```python
from build123d import *

# Parameters (mm, degrees)
BOSS_EXTRUDE1_DEPTH            = 25
SKETCH2_R                      = 2.6
SKETCH2_R_2                    = 1.55
BOSS_EXTRUDE3_DEPTH            = 5
CUT_EXTRUDE1_REACH             = 98.604
CUT_EXTRUDE1_DIRECTION_2_DEPTH = 97.603907966
CUT_EXTRUDE2_REACH             = 98.604
CUT_EXTRUDE2_DIRECTION_2_DEPTH = 97.603907966
FILLET1_R                      = 2
SKETCH6_R                      = 2.6
BOSS_EXTRUDE4_DEPTH            = 1


with BuildPart() as part:
    # Sketch1 → Boss-Extrude1 (new body)
    with BuildSketch(Plane(origin=(0, 0, 0), x_dir=(1, 0, 0), z_dir=(0, 1, 0))):
        Polygon((-13.5, 0), (0, 83.718518379), (13.5, 0), (14.487246657, 0.15919811), (0, 90), (-14.487246657, 0.15919811), align=None)
    extrude(amount=BOSS_EXTRUDE1_DEPTH)

    # Sketch2 → Boss-Extrude3 (add)
    # profile 1 of 8: a face of its own
    with BuildSketch(Plane(origin=(0, 0, 0), x_dir=(1, 0, 0), z_dir=(0, 1, 0))):
        with Locations((11.920405349, -0.254716975)):
            Circle(SKETCH2_R)
        with Locations(Location((11.920405349, -0.254716975, 0), (0, 0, 270))):
            Circle(SKETCH2_R_2, mode=Mode.SUBTRACT)
    # profile 2 of 8: a face of its own
    with BuildSketch(Plane(origin=(0, 0, 0), x_dir=(1, 0, 0), z_dir=(0, 1, 0))):
        with Locations((9.373235594, 15.541229537)):
            Circle(SKETCH2_R)
        with Locations(Location((9.373235594, 15.541229537, 0), (0, 0, 270))):
            Circle(SKETCH2_R_2, mode=Mode.SUBTRACT)
    # profile 3 of 8: a face of its own
    with BuildSketch(Plane(origin=(0, 0, 0), x_dir=(1, 0, 0), z_dir=(0, 1, 0))):
        with Locations((6.826065839, 31.33717605)):
            Circle(SKETCH2_R)
        with Locations(Location((6.826065839, 31.33717605, 0), (0, 0, 270))):
            Circle(SKETCH2_R_2, mode=Mode.SUBTRACT)
    # profile 4 of 8: a face of its own
    with BuildSketch(Plane(origin=(0, 0, 0), x_dir=(1, 0, 0), z_dir=(0, 1, 0))):
        with Locations((4.278896085, 47.133122563)):
            Circle(SKETCH2_R)
        with Locations(Location((4.278896085, 47.133122563, 0), (0, 0, 270))):
            Circle(SKETCH2_R_2, mode=Mode.SUBTRACT)
    # profile 5 of 8: a face of its own
    with BuildSketch(Plane(origin=(0, 0, 0), x_dir=(1, 0, 0), z_dir=(0, 1, 0))):
        with Locations((-4.278896085, 47.133122563)):
            Circle(SKETCH2_R)
        with Locations(Location((-4.278896085, 47.133122563, 0), (0, 0, 90))):
            Circle(SKETCH2_R_2, mode=Mode.SUBTRACT)
    # profile 6 of 8: a face of its own
    with BuildSketch(Plane(origin=(0, 0, 0), x_dir=(1, 0, 0), z_dir=(0, 1, 0))):
        with Locations((-6.826065839, 31.33717605)):
            Circle(SKETCH2_R)
        with Locations(Location((-6.826065839, 31.33717605, 0), (0, 0, 90))):
            Circle(SKETCH2_R_2, mode=Mode.SUBTRACT)
    # profile 7 of 8: a face of its own
    with BuildSketch(Plane(origin=(0, 0, 0), x_dir=(1, 0, 0), z_dir=(0, 1, 0))):
        with Locations((-9.373235594, 15.541229537)):
            Circle(SKETCH2_R)
        with Locations(Location((-9.373235594, 15.541229537, 0), (0, 0, 90))):
            Circle(SKETCH2_R_2, mode=Mode.SUBTRACT)
    # profile 8 of 8: a face of its own
    with BuildSketch(Plane(origin=(0, 0, 0), x_dir=(1, 0, 0), z_dir=(0, 1, 0))):
        with Locations((-11.920405349, -0.254716975)):
            Circle(SKETCH2_R)
        with Locations(Location((-11.920405349, -0.254716975, 0), (0, 0, 90))):
            Circle(SKETCH2_R_2, mode=Mode.SUBTRACT)
    boss_extrude3 = extrude(amount=BOSS_EXTRUDE3_DEPTH)

    # Cut-Extrude1: up to this face of the body (flat: up to its plane)
    cut_extrude1_end = Plane(part.part.faces().sort_by_distance((-6.667350715, 12.850191169, -42.371798131))[0])
    # Sketch4 → Cut-Extrude1 (cut, up to the picked face)
    with BuildSketch(Plane(origin=(0.342144515, 0, 2.121765321), x_dir=(0.9872466570606503, 0, -0.1591981096702188), z_dir=(0.1591981096702188, 0, 0.9872466570606503)), mode=Mode.PRIVATE) as cut_extrude1_sk1:
        Polygon((13.32782987, 5), (9.12782987, 5), (9.12782987, 1.475781549), align=None)
    cut_extrude1_tool1 = split(extrude(cut_extrude1_sk1.sketch, amount=-CUT_EXTRUDE1_REACH, mode=Mode.PRIVATE), bisect_by=cut_extrude1_end, keep=Keep.BOTH, mode=Mode.PRIVATE)
    cut_extrude1 = cut_extrude1_tool1.solids().sort_by(Axis((10.735709, 3.825261, 0.445755), (-0.1591981096702188, 0, -0.9872466570606503)))[0]
    add(cut_extrude1, mode=Mode.SUBTRACT)

    # Sketch4 → Cut-Extrude1 direction 2 (cut)
    with BuildSketch(Plane(origin=(0.342144515, 0, 2.121765321), x_dir=(0.9872466570606503, 0, -0.1591981096702188), z_dir=(0.1591981096702188, 0, 0.9872466570606503))):
        Polygon((13.32782987, 5), (9.12782987, 5), (9.12782987, 1.475781549), align=None)
    cut_extrude1_direction_2 = extrude(amount=CUT_EXTRUDE1_DIRECTION_2_DEPTH, mode=Mode.SUBTRACT)

    # Cut-Extrude2: up to this face of the body (flat: up to its plane)
    cut_extrude2_end = Plane(part.part.faces().sort_by_distance((6.667350715, 12.850191169, -42.371798131))[0])
    # Sketch5 → Cut-Extrude2 (cut, up to the picked face)
    with BuildSketch(Plane(origin=(-0.342144515, 0, 2.121765321), x_dir=(0.9872466570606502, 0, 0.15919810967021986), z_dir=(-0.15919810967021986, 0, 0.9872466570606502)), mode=Mode.PRIVATE) as cut_extrude2_sk1:
        Polygon((-9.12782987, 5), (-9.12782987, 1.475781549), (-13.32782987, 5), align=None)
    cut_extrude2_tool1 = split(extrude(cut_extrude2_sk1.sketch, amount=-CUT_EXTRUDE2_REACH, mode=Mode.PRIVATE), bisect_by=cut_extrude2_end, keep=Keep.BOTH, mode=Mode.PRIVATE)
    cut_extrude2 = cut_extrude2_tool1.solids().sort_by(Axis((-10.735709, 3.825261, 0.445755), (0.15919810967021986, 0, -0.9872466570606502)))[0]
    add(cut_extrude2, mode=Mode.SUBTRACT)

    # Sketch5 → Cut-Extrude2 direction 2 (cut)
    with BuildSketch(Plane(origin=(-0.342144515, 0, 2.121765321), x_dir=(0.9872466570606502, 0, 0.15919810967021986), z_dir=(-0.15919810967021986, 0, 0.9872466570606502))):
        Polygon((-9.12782987, 5), (-9.12782987, 1.475781549), (-13.32782987, 5), align=None)
    cut_extrude2_direction_2 = extrude(amount=CUT_EXTRUDE2_DIRECTION_2_DEPTH, mode=Mode.SUBTRACT)

    # Mirror2: Boss-Extrude3, Cut-Extrude1, Cut-Extrude1 direction 2, Cut-Extrude2, Cut-Extrude2 direction 2 across plane
    add(boss_extrude3.mirror(Plane.ZX.offset(12.5)))
    add(cut_extrude1.mirror(Plane.ZX.offset(12.5)), mode=Mode.SUBTRACT)
    add(cut_extrude1_direction_2.mirror(Plane.ZX.offset(12.5)), mode=Mode.SUBTRACT)
    add(cut_extrude2.mirror(Plane.ZX.offset(12.5)), mode=Mode.SUBTRACT)
    add(cut_extrude2_direction_2.mirror(Plane.ZX.offset(12.5)), mode=Mode.SUBTRACT)

    # Fillet1
    # the kernel refuses this fillet: 2 mm, written as the material it adds along each edge
    with BuildSketch(Plane(origin=(-19.423479942, 5, -0.955188658), x_dir=(-0.15919810967021975, 0, 0.9872466570606501), z_dir=(0.9872466570606501, 0, 0.15919810967021975))) as fillet1_piece_1_section:
        with BuildLine():
            CenterArc((FILLET1_R, -FILLET1_R), FILLET1_R, 90, 90)
            Line((0, -FILLET1_R), (0, 0))
            Line((0, 0), (FILLET1_R, 0))
        make_face()
    fillet1_piece_1 = extrude(amount=6, mode=Mode.PRIVATE)
    fillet1_piece_1 = fillet1_piece_1 & Plane(origin=(-11.920405349, 5.222362792, 0.254716975), x_dir=(1, 0, 0), z_dir=(0, -1, 0)) * Cylinder(2.6, 21, mode=Mode.PRIVATE)
    add(fillet1_piece_1)
    with BuildSketch(Plane(origin=(13.5, 5, 0), x_dir=(0, 1, 0), z_dir=(0.9872466570606502, 0, -0.15919810967021866))) as fillet1_piece_2_section:
        with BuildLine():
            CenterArc((FILLET1_R, FILLET1_R), FILLET1_R, 180, 90)
            Line((0, FILLET1_R), (0, 0))
            Line((0, 0), (FILLET1_R, 0))
        make_face()
    fillet1_piece_2 = extrude(amount=6, mode=Mode.PRIVATE)
    fillet1_piece_2 = fillet1_piece_2 & Plane(origin=(11.920405349, 5.699977741, 0.254716975), x_dir=(1, 0, 0), z_dir=(0, -1, 0)) * Cylinder(2.6, 20, mode=Mode.PRIVATE)
    add(fillet1_piece_2)
    with BuildSketch(Plane(origin=(13.5, 20, 0), x_dir=(0, -1, 0), z_dir=(0.9872466570606502, 0, -0.15919810967021866))) as fillet1_piece_3_section:
        with BuildLine():
            CenterArc((FILLET1_R, -FILLET1_R), FILLET1_R, 90, 90)
            Line((0, -FILLET1_R), (0, 0))
            Line((0, 0), (FILLET1_R, 0))
        make_face()
    fillet1_piece_3 = extrude(amount=6, mode=Mode.PRIVATE)
    fillet1_piece_3 = fillet1_piece_3 & Plane(origin=(11.920405349, 19.300022259, 0.254716975), x_dir=(1, 0, 0), z_dir=(0, 1, 0)) * Cylinder(2.6, 20, mode=Mode.PRIVATE)
    add(fillet1_piece_3)
    with BuildSketch(Plane(origin=(-19.423479942, 20, -0.955188658), x_dir=(0, -1, 0), z_dir=(0.9872466570606501, 0, 0.15919810967021975))) as fillet1_piece_4_section:
        with BuildLine():
            CenterArc((FILLET1_R, -FILLET1_R), FILLET1_R, 90, 90)
            Line((0, -FILLET1_R), (0, 0))
            Line((0, 0), (FILLET1_R, 0))
        make_face()
    fillet1_piece_4 = extrude(amount=6, mode=Mode.PRIVATE)
    fillet1_piece_4 = fillet1_piece_4 & Plane(origin=(-11.920405349, 19.777637105, 0.254716975), x_dir=(1, 0, 0), z_dir=(0, 1, 0)) * Cylinder(2.6, 21, mode=Mode.PRIVATE)
    add(fillet1_piece_4)

    # Sketch6 → Boss-Extrude4 (add)
    with BuildSketch(Plane.XZ):
        with Locations((11.920405349, 0.254716975)):
            Circle(SKETCH6_R)
        with Locations((9.373235594, -15.541229537)):
            Circle(SKETCH6_R)
        with Locations((6.826065839, -31.33717605)):
            Circle(SKETCH6_R)
        with Locations((4.278896085, -47.133122563)):
            Circle(SKETCH6_R)
        with Locations((-4.278896085, -47.133122563)):
            Circle(SKETCH6_R)
        with Locations((-6.826065839, -31.33717605)):
            Circle(SKETCH6_R)
        with Locations((-9.373235594, -15.541229537)):
            Circle(SKETCH6_R)
        with Locations((-11.920405349, 0.254716975)):
            Circle(SKETCH6_R)
    extrude(amount=-BOSS_EXTRUDE4_DEPTH)


solid = part.part
```
Geometry: final body of the model. Coordinates: model frame, mm. A direction names the side the tool comes from. Coordinates: 2 decimals unless noted, no trailing zeros. Order: outer loops, then holes, each group sorted by start corner. A loop starts at its lowest first (then second) coordinate and runs counter-clockwise, first axis right, second up. Notation, with made-up numbers: (-38.75, 2.5) -> (-3.75, 2.5) arc R16 cw to (-3.75, 13.5) -> close; hole circle Ø11 at (-13.75, -2). An arc over 180 degrees is marked (long way). Answer in a Markdown table with one row per item.
Item 1: Contact query for flat-ended pins moving along their axis: P1, Ø1.5, axis at y = 17.5, z = -14, coming from the -X side; P2, Ø4, axis at y = 5, z = -59.5, coming from the -X side; P3, Ø0.9, axis at x = 12, z = -0.5, coming from the +Y side. Output: stop coordinate, or through.
Return value:
| item | result |
|---|---|
| P1 | stops at x = -12.38 |
| P2 | stops at x = -5.24 |
| P3 | stops at y = 1 |
Item 2: Section B-B on y = 13. Output: boundary loops of the cut face in (x, z), plus the area to 3 significant figures.
Return value:
| item | result |
|---|---|
| outline | (-14.49, -0.16) -> (0, -90) -> (14.49, -0.16) -> (13.5, 0) -> (0, -83.72) -> (-13.5, 0) -> close |
| area | 176 mm² |
Item 3: Ray query, L1, parallel to Y at x = -5.25, z = -33; L2, parallel to Y at x = 4.75, z = -31; L3, parallel to X at y = 16, z = -2.5. Return the intervals inside material, ascending.
Return value:
| item | result |
|---|---|
| L1 | y = 0 to 2.57, 22.43 to 25 |
| L2 | y = 0 to 1.89, 23.11 to 25 |
| L3 | x = -14.11 to -13.1, 13.1 to 14.11 |
Item 4: Section A-A on z = -42.5. Output: boundary loops of the cut face in (x, y), plus the area to 3 significant figures.
Return value:
| item | result |
|---|---|
| outline | (-7.66, 0) -> (-6.65, 0) -> (-6.65, 25) -> (-7.66, 25) -> close; (6.65, 0) -> (7.66, 0) -> (7.66, 25) -> (6.65, 25) -> close |
| area | 50.6 mm² |
Item 5: Draft query along Y for faces 4 (the cylindrical face through (10.91, 23.1, -15.74)), 5 (the flat face through (-5.204, 2.43, -32.209)), 6 (the flat face through (-4, 1, -47)). Return one class per face: released by +Y, released by -Y, zero draft, split by the parting line, or undercut.
Return value:
| item | result |
|---|---|
| face 4 | zero draft |
| face 5 | undercut |
| face 6 | released by +Y |
Item 6: Access query for faces 1 (the flat face through (7.75, 2.43, -16.41)), 2 (the cylindrical face through (10.91, 2.52, -15.74)), 3 (the cylindrical face through (-13.95, 5.83, 0.31)). Directions: +Z, -Z, +X, -X, +Y, -Y. A direction counts if a zero-diameter tool reaches every point of the face in a straight line with its end or side. Return the directions, or none.
Return value:
| item | result |
|---|---|
| face 1 | +Z |
| face 2 | +Y |
| face 3 | +Z, -X |
Item 7: Section C-C on y = 6. Output: boundary loops of the cut face in (x, z), plus the area to 3 significant figures.
Return value:
| item | result |
|---|---|
| outline | (-14.52, 0.11) arc R2.6 ccw to (-14.49, -0.16) -> (0, -90) -> (14.49, -0.16) arc R2.6 ccw to (14.52, 0.11) -> (13.54, 0.26) -> (0, -83.72) -> (-13.54, 0.26) -> close |
| area | 176 mm² |
